Design review of the part shown in the three views and the two pictorial views. Dimensions are in mm from the part's minimum x, y and z. A direction names the side the tool comes from. Round coordinates to 2 decimals unless told otherwise and drop trailing zeros. Order: outer loops, then holes, each group sorted by start corner. A loop starts at its lowest first (then second) coordinate and runs counter-clockwise, first axis right, second up.
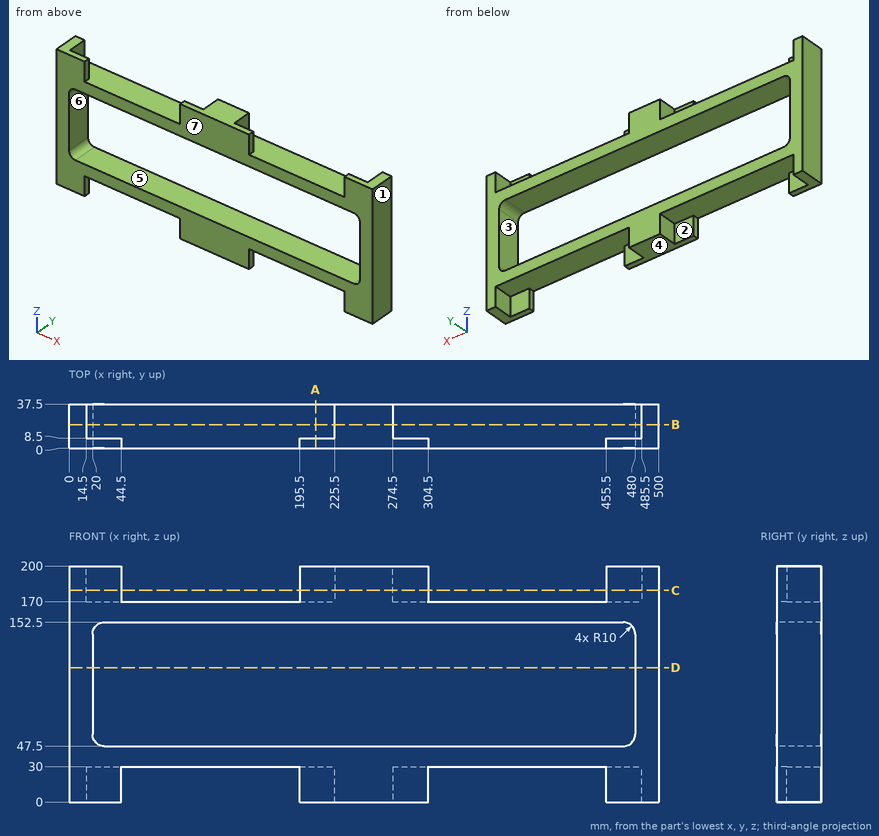
1) To check wall thickness, follow line 1 along X through (y, z) = (11, 11); line 2 along Z through (x, y) = (32.5, 16.5); line 3 along X through (y, z) = (15, 71). State the ranges of each line that lie inside material, in increasing order.
Results:
line 1: x = 0 to 14.5, 225.5 to 274.5, 485.5 to 500
line 2: z = 30 to 47.5, 152.5 to 170
line 3: x = 0 to 20, 480 to 500
2) Take a section at B-B on y = 20. Give the boundary of the cut face in (x, z), plus the area to 3 significant figures.
Results:
outline: (0, 0) - (14.5, 0) - (14.5, 30) - (225.5, 30) - (225.5, 0) - (274.5, 0) - (274.5, 30) - (485.5, 30) - (485.5, 0) - (500, 0) - (500, 200) - (485.5, 200) - (485.5, 170) - (274.5, 170) - (274.5, 200) - (225.5, 200) - (225.5, 170) - (14.5, 170) - (14.5, 200) - (0, 200) - close; hole (20, 57.5) arc R10 ccw to (30, 47.5) - (470, 47.5) arc R10 ccw to (480, 57.5) - (480, 142.5) arc R10 ccw to (470, 152.5) - (30, 152.5) arc R10 ccw to (20, 142.5) - close
area: 26,500 mm2
3) Clearance check with flat-ended pins moving along their axes: P1, Ø3, axis at x = 138, y = 5, coming from the +Z side; P2, Ø19, axis at x = 347, y = 17, coming from the -Z side; P3, Ø15, axis at x = 471, z = 180.5, coming from the +Y side; P4, Ø12, axis at y = 22.5, z = 145.5, coming from the -X side. State where each tip first meets the part, or that it passes through.
Results:
P1: stops at z = 170
P2: stops at z = 30
P3: stops at y = 8.5
P4: stops at x = 0
4) For the marked faces 1, 2 and 3, list the 3-axis set-ups (+Z, -Z, +X, -X, +Y, -Y) from which the entire face can be reached by the end or side of a thin tool; tool diameter is ignored.
Results:
face 1: +Z, -Z, +X, +Y, -Y
face 2: -Z, +Y
face 3: +Y, -Y
5) Take a section at C-C on z = 179.5. Give the boundary of the cut face in (x, y), plus the area to 4 significant figures.
Results:
outline: (0, 0) - (44.5, 0) - (44.5, 8.5) - (14.5, 8.5) - (14.5, 37.5) - (0, 37.5) - close; (195.5, 0) - (304.5, 0) - (304.5, 8.5) - (274.5, 8.5) - (274.5, 37.5) - (225.5, 37.5) - (225.5, 8.5) - (195.5, 8.5) - close; (455.5, 0) - (500, 0) - (500, 37.5) - (485.5, 37.5) - (485.5, 8.5) - (455.5, 8.5) - close
area: 3,945 mm2
6) Take a section at A-A on x = 209. Give the boundary of the cut face in (y, z), plus the area to 3 significant figures.
Results:
outline: (0, 0) - (8.5, 0) - (8.5, 30) - (37.5, 30) - (37.5, 47.5) - (0, 47.5) - close; (0, 152.5) - (37.5, 152.5) - (37.5, 170) - (8.5, 170) - (8.5, 200) - (0, 200) - close
area: 1,820 mm2
7) Take a section at D-D on z = 114. Give the boundary of the cut face in (x, y), plus the area to 3 significant figures.
Results:
outline: (0, 0) - (20, 0) - (20, 37.5) - (0, 37.5) - close; (480, 0) - (500, 0) - (500, 37.5) - (480, 37.5) - close
area: 1,500 mm2
8) The part is to be moulded in two halves that separate along Z. For the marked faces 4, 5, 6 and 7, say which applies: released by +Z, released by -Z, zero draft, split by the parting line, or undercut.
Results:
face 4: released by -Z
face 5: undercut
face 6: undercut
face 7: zero draft
